Read the model definition and answer for the solid it produces. Units are mm, in the model's axes. A direction names the side the tool comes from. Give positions to 0.01 mm unless a question says otherwise; leave off trailing zeros. Order: outer loops, then holes, each group sorted by start corner. A loop starts at its lowest first (then second) coordinate and runs counter-clockwise, first axis right, second up. Notation, with made-up numbers: (-14.5, -14.5) - (29.5, -14.5) arc R14 ccw to (29.5, 4.5) - close; hole circle Ø11 at (0.5, 77.5). An arc over 180 degrees is marked (long way). Write item = value, one per line.
```python
from build123d import *

# Parameters (mm, degrees)
F0_R     = 46.9907893429
F0_R_2   = 32.2922795361
F1_DEPTH = 60
F3_DEPTH = 15
F5_DEPTH = 7.5


with BuildPart() as f1:
    # F0 (on Top) → F1 (new body)
    with BuildSketch(Plane.XY):
        with Locations((50.2018332481, 0)):
            Circle(F0_R)
        with Locations((50.2018332481, 0)):
            Circle(F0_R_2, mode=Mode.SUBTRACT)
    extrude(amount=F1_DEPTH)

    # F2 (on face) → F3 (join)
    with BuildSketch(Plane(origin=(0, 0, 0), x_dir=(1, 0, 0), z_dir=(0, 0, -1))):
        with BuildLine():
            ThreePointArc((44.7961655187, -46.6788286), (3.2110439053, 0), (44.7961655187, 46.6788286))
            Line((44.7961655187, 46.6788286), (-54.8171773669, 46.6788286))
            Line((-54.8171773669, 46.6788286), (-54.8171773669, -46.6788286))
            Line((-54.8171773669, -46.6788286), (44.7961655187, -46.6788286))
        make_face()
    extrude(amount=-F3_DEPTH)

    # F4 (on Front) → F5 (join, symmetric)
    with BuildSketch(Plane.XZ):
        Polygon((4.0778061375, 54.1363731027), (-44.1848946292, 14.6238496527), (4.0778061375, 14.6238496527), align=None)
    extrude(amount=F5_DEPTH, both=True)


solid = f1.part
```
1. Section D-D (y = 29) is taken. Determine the outline of the cut face in (x, z).
Recorded:
outline = (-54.82, 0) - (36, 0) - (36, 60) - (13.23, 60) - (13.23, 15) - (-54.82, 15) - close; (64.41, 0) - (87.18, 0) - (87.18, 60) - (64.41, 60) - close
2. Flat-ended cylindrical pins translate along their axes: pin 1 (16.5 mm diameter, centred on x = -28, z = 11, fed in from +Y); pin 2 (5 mm diameter, centred on x = 64, z = 44.5, fed in from -Y); pin 3 (3 mm diameter, centred on x = 52, z = 12.5, fed in from -Y); pin 4 (12 mm diameter, centred on x = 8, z = 8, fed in from -Y). Find the tip coordinate at first contact, or state that the pin passes through.
Recorded:
pin_1 = 46.68
pin_2 = -45.61
pin_3 = -46.99
pin_4 = -46.68
3. For faces 1 (the face through (-10, 7.5, 26)), 2 (the face through (-10, -7.5, 26)), 3 (the face through (95.023, 14.115, 29.58)), determine the directions among +Z, -Z, +X, -X, +Y, -Y from which every point of the face is accessible in a straight line to the end or side of a thin tool.
Recorded:
face_1 = +Z, -X, +Y
face_2 = +Z, -X, -Y
face_3 = +Z
4. Straight lines are drawn through the part: L1, parallel to Y at x = 66.5, z = 49; L2, parallel to Z at x = 1, y = -27.5; L3, parallel to X at y = 12, z = 50.5. For each, find the intervals that lie inside material, in ascending order. Write a range as [from, to].
Recorded:
L1 = [-44.07, -27.88], [27.88, 44.07]
L2 = [0, 15]
L3 = [4.77, 20.22], [80.18, 95.63]
5. Determine the mould class of faces 4 (the face through (-19.623, -0.105, 34.732)), 5 (the face through (80.03, -12.37, 29.58)), 6 (the face through (81, 11, 60)) for opening direction X: +X half, -X half, draft (parallel to the pull), parting line (faces both ways), or undercut.
Recorded:
face_4 = -X half
face_5 = undercut
face_6 = draft
6. Section C-C (z = 21.5) is taken. Determine the outline of the cut face in (x, y).
Recorded:
outline = (-35.79, -7.5) - (3.81, -7.5) arc R46.99 ccw (long way) to (3.81, 7.5) - (-35.79, 7.5) - close; hole circle Ø64.58 at (50.2, 0)
7. Section A-A (y = 4) is taken. Determine the outline of the cut face in (x, z).
Recorded:
outline = (-54.82, 0) - (18.16, 0) - (18.16, 60) - (3.38, 60) - (3.38, 53.57) - (-43.73, 15) - (-54.82, 15) - close; (82.25, 0) - (97.02, 0) - (97.02, 60) - (82.25, 60) - close
8. Section B-B (x = 37.5) is taken. Determine the outline of the cut face in (y, z), and give its area (3 significant figures).
Recorded:
outline = (-46.68, 0) - (-29.69, 0) - (-29.69, 60) - (-45.24, 60) - (-45.24, 15) - (-46.68, 15) - close; (29.69, 0) - (46.68, 0) - (46.68, 15) - (45.24, 15) - (45.24, 60) - (29.69, 60) - close
area = 1,910 mm^2
